from build123d import *

# Parameters (mm, degrees)
SKETCH1_W           = 63
SKETCH1_H           = 36
SKETCH1_W_2         = 57
SKETCH1_H_2         = 30
BOSS_EXTRUDE1_DEPTH = 98
SKETCH2_W           = 57
SKETCH2_H           = 30
BOSS_EXTRUDE2_DEPTH = 3


with BuildPart() as part:
    # Sketch1 → Boss-Extrude1 (new body)
    with BuildSketch(Plane.XY):
        Rectangle(SKETCH1_W, SKETCH1_H)
        Rectangle(SKETCH1_W_2, SKETCH1_H_2, mode=Mode.SUBTRACT)
    extrude(amount=BOSS_EXTRUDE1_DEPTH)

    # Sketch2 → Boss-Extrude2 (add)
    with BuildSketch(Plane(origin=(0, 0, 0), x_dir=(-1, 0, 0), z_dir=(0, 0, -1))):
        Rectangle(SKETCH2_W, SKETCH2_H)
    extrude(amount=-BOSS_EXTRUDE2_DEPTH)


solid = part.part
Model file for the job. Use its own axes, mm. A direction names the side the tool comes from. Give positions to 0.01 mm unless a question says otherwise; leave off trailing zeros. Order: outer loops, then holes, each group sorted by start corner. A loop starts at its lowest first (then second) coordinate and runs counter-clockwise, first axis right, second up. Notation, with made-up numbers: (-37, 18) - (9, 18) arc R13 cw to (9, 31) - close; hole circle Ø5 at (21.5, 65.25). An arc over 180 degrees is marked (long way). One line per item, written item: value.
Item 1: Tool access for faces 1 (the flat face through (31.5, 0, 48)), 2 (the flat face through (-28.5, 0, 50)): list every direction of +Z, -Z, +X, -X, +Y, -Y with a clear straight run to the whole face (end or side of a thin tool).
Response values:
face 1: +Z, -Z, +X, +Y, -Y
face 2: +Z
Item 2: Two-plate mould, pull along Y, no slides. Class faces 3 (the flat face through (0, -18, 48)), 4 (the flat face through (-2, -16, 98)), 5 (the flat face through (0, -15, 50)): released by +Y, released by -Y, zero draft, split by the parting line, or undercut.
Response values:
face 3: released by -Y
face 4: zero draft
face 5: undercut
Item 3: Wall check: line 1 (Y direction, x = 4, z = 48); line 2 (X direction, y = -2, z = 21); line 3 (Z direction, x = 24.5, y = -4.5). Give the ranges that are in metal, low to high.
Response values:
line 1: -18 to -15, 15 to 18
line 2: -31.5 to -28.5, 28.5 to 31.5
line 3: 0 to 3
Item 4: Slice it at B-B (x = -21). List the corners of the cut face in (y, z).
Response values:
outline: (-18, 0) - (18, 0) - (18, 98) - (15, 98) - (15, 3) - (-15, 3) - (-15, 98) - (-18, 98) - close
Item 5: Slice it at A-A (z = 47.5). List the corners of the cut face in (x, y), then the cut area to 3 significant figures.
Response values:
outline: (-31.5, -18) - (31.5, -18) - (31.5, 18) - (-31.5, 18) - close; hole (-28.5, -15) - (28.5, -15) - (28.5, 15) - (-28.5, 15) - close
area: 558 mm2
Item 6: Slice it at C-C (y = 14). List the corners of the cut face in (x, z).
Response values:
outline: (-31.5, 0) - (31.5, 0) - (31.5, 98) - (28.5, 98) - (28.5, 3) - (-28.5, 3) - (-28.5, 98) - (-31.5, 98) - close
